Geometry: final body of the model. Coordinates: model frame, mm. A direction names the side the tool comes from. Round coordinates to 2 decimals unless told otherwise and drop trailing zeros. Write each loop counter-clockwise with the first axis right and the second up, starting at its lowest first coordinate (ties: lowest second). Pieces come first, ordered by that corner, then holes. Notation, with made-up numbers: (84.5, 2.25) -> (116.5, 2.25) arc R10 cw to (116.5, 7.25) -> close; hole circle Ø3 at (-37, -24.75). An arc over 180 degrees is marked (long way). Use one line per item in the form item = value. Start each with the question number.
1. Cut plane C-C, the plane x = -10.65. Return the cut outline in (y, z).
2. Draft query along Y for faces 1 (the face through (9.65, 7.24, 17.37)), 2 (the face through (0, 9.3, 17)), 3 (the face through (0, 0, 0)), 4 (the face through (0, 16, 18)). Return one class per face: pulls with the +Y half, pulls with the -Y half, needs draft (parallel to the pull), parting line crosses it, or undercut.
3. Line query: L1, parallel to X at y = 7.25, z = -10; L2, parallel to Z at x = 8.5, y = 21.75; L3, parallel to Y at x = -10.65, z = 19.55. Output: solid intervals per line, ascending.
4. Pin query (flat end, axial travel): pin 1 Ø2.5 at (x, y) = (-10.65, 7.2) entering from +Z; pin 2 Ø3 at (x, z) = (-5.5, -4.5) entering from +Y; pin 3 Ø1.2 at (x, y) = (-11.5, 10.5) entering from -Z. Return the tip coordinate at first contact, or that it passes through.
5. Cut plane A-A, the plane y = 7.2. Return the cut outline in (x, z).
6. Reachability of faces 5 (the face through (9.49, 12.686, -18.817)), 6 (the face through (-9.696, 7.5, 17.368)), 7 (the face through (0, 14, -17.2)) from +Z, -Z, +X, -X, +Y, -Y: full face, straight path, thin tool, end or side. Return the list, or none.
7. Cut plane B-B, the plane z = -13. Return the cut outline in (x, y), plus the area to 3 significant figures.
8. Cut plane D-D, the plane y = 18.5. Return the cut outline in (x, z), plus the area to 3 significant figures.
```python
from build123d import *

# Parameters (mm, degrees)
SKETCH_3_W           = 36
SKETCH_3_H           = 50
EXTRUDE_1_DEPTH      = 24
SKETCH_4_W           = 24.8
SKETCH_4_H           = 31.8
CUT_EXTRUDE_1_DEPTH  = 19.7
SKETCH_5_W           = 14
SKETCH_5_H           = 2.2
CUT_EXTRUDE_3_DEPTH  = 19.7
SKETCH_6_W           = 18.5
SKETCH_6_H           = 3.8
CUT_EXTRUDE_4_DEPTH  = 14.7
SKETCH_7_W           = 24.8
SKETCH_7_H           = 24.280407208
CUT_EXTRUDE_5_DEPTH  = 2
SKETCH_8_R           = 2
CUT_EXTRUDE_6_DEPTH  = 6.4
SKETCH_9_R           = 1
CUT_EXTRUDE_7_DEPTH  = 6.4
SKETCH_10_R          = 2
CUT_EXTRUDE_8_DEPTH  = 7.4
SKETCH_11_R          = 1
CUT_EXTRUDE_9_DEPTH  = 7.4
SKETCH_14_W          = 47.693248889
SKETCH_14_H          = 41.94352182
CUT_EXTRUDE_12_DEPTH = 4
SKETCH_16_W          = 69.166934332
SKETCH_16_H          = 39.422219991
CUT_EXTRUDE_13_DEPTH = 5
CUT_EXTRUDE_17_DEPTH = 19.7
SKETCH_19_W          = 18.9
SKETCH_19_H          = 2.1
CUT_EXTRUDE_18_DEPTH = 12.7
SKETCH_20_W          = 25.2
SKETCH_20_H          = 38.217614171
CUT_EXTRUDE_19_DEPTH = 2


with BuildPart() as part:
    # 草图3 → 凸台-拉伸1 (new body)
    with BuildSketch(Plane(origin=(0, 0, 0), x_dir=(1, 0, 0), z_dir=(0, 1, 0))):
        Rectangle(SKETCH_3_W, SKETCH_3_H)
    extrude(amount=EXTRUDE_1_DEPTH)

    # 草图4 → 切除-拉伸1 (cut)
    with BuildSketch(Plane(origin=(0, 24, 0), x_dir=(1, 0, 0), z_dir=(0, 1, 0))):
        Rectangle(SKETCH_4_W, SKETCH_4_H)
    extrude(amount=-CUT_EXTRUDE_1_DEPTH, mode=Mode.SUBTRACT)

    # 草图5 → 切除-拉伸3 (cut)
    with BuildSketch(Plane(origin=(0, 24, 0), x_dir=(1, 0, 0), z_dir=(0, 1, 0))):
        with Locations((0, 15.9)):
            Rectangle(SKETCH_5_W, SKETCH_5_H)
    extrude(amount=-CUT_EXTRUDE_3_DEPTH, mode=Mode.SUBTRACT)

    # 草图6 → 切除-拉伸4 (cut)
    with BuildSketch(Plane(origin=(0, 24, 0), x_dir=(1, 0, 0), z_dir=(0, 1, 0))):
        with Locations((0, -15.9)):
            Rectangle(SKETCH_6_W, SKETCH_6_H)
    extrude(amount=-CUT_EXTRUDE_4_DEPTH, mode=Mode.SUBTRACT)

    # 草图7 → 切除-拉伸5 (cut)
    with BuildSketch(Plane(origin=(0, 24, 0), x_dir=(1, 0, 0), z_dir=(0, 1, 0))):
        with Locations((0, -25)):
            Rectangle(SKETCH_7_W, SKETCH_7_H)
    extrude(amount=-CUT_EXTRUDE_5_DEPTH, mode=Mode.SUBTRACT)

    # 草图8 → 切除-拉伸6 (cut)
    with BuildSketch(Plane.XY.offset(25)):
        with Locations((10.65, 7.2)):
            Circle(SKETCH_8_R)
        with Locations((-10.65, 7.2)):
            Circle(SKETCH_8_R)
    extrude(amount=-CUT_EXTRUDE_6_DEPTH, mode=Mode.SUBTRACT)

    # 草图9 → 切除-拉伸7 (cut)
    with BuildSketch(Plane.XY.offset(18.6)):
        with Locations((10.65, 7.2)):
            Circle(SKETCH_9_R)
        with Locations((-10.65, 7.2)):
            Circle(SKETCH_9_R)
    extrude(amount=-CUT_EXTRUDE_7_DEPTH, mode=Mode.SUBTRACT)

    # 草图10 → 切除-拉伸8 (cut)
    with BuildSketch(Plane(origin=(0, 0, -25), x_dir=(-1, 0, 0), z_dir=(0, 0, -1))):
        with Locations((-10.565, 11)):
            Circle(SKETCH_10_R)
        with Locations((10.56, 11)):
            Circle(SKETCH_10_R)
    extrude(amount=-CUT_EXTRUDE_8_DEPTH, mode=Mode.SUBTRACT)

    # 草图11 → 切除-拉伸9 (cut)
    with BuildSketch(Plane(origin=(0, 0, -17.6), x_dir=(-1, 0, 0), z_dir=(0, 0, -1))):
        with Locations((10.56, 11)):
            Circle(SKETCH_11_R)
        with Locations((-10.565, 11)):
            Circle(SKETCH_11_R)
    extrude(amount=-CUT_EXTRUDE_9_DEPTH, mode=Mode.SUBTRACT)

    # 草图14 → 切除-拉伸12 (cut)
    with BuildSketch(Plane.XY.offset(25)):
        with Locations((-2.653720185, 12.393348568)):
            Rectangle(SKETCH_14_W, SKETCH_14_H)
    extrude(amount=-CUT_EXTRUDE_12_DEPTH, mode=Mode.SUBTRACT)

    # 草图16 → 切除-拉伸13 (cut)
    with BuildSketch(Plane(origin=(0, 0, -25), x_dir=(-1, 0, 0), z_dir=(0, 0, -1))):
        with Locations((0.858826259, 12.588310345)):
            Rectangle(SKETCH_16_W, SKETCH_16_H)
    extrude(amount=-CUT_EXTRUDE_13_DEPTH, mode=Mode.SUBTRACT)

    # 草图18 → 切除-拉伸17 (cut)
    with BuildSketch(Plane(origin=(0, 24, 0), x_dir=(1, 0, 0), z_dir=(0, 1, 0))):
        Polygon((-12.6, -16.1), (12.6, -16.1), (12.6, 16.1), (7.2, 16.1), (7.2, 17.2), (-7.2, 17.2), (-7.2, 16.1), (-12.6, 16.1), align=None)
    extrude(amount=-CUT_EXTRUDE_17_DEPTH, mode=Mode.SUBTRACT)

    # 草图19 → 切除-拉伸18 (cut)
    with BuildSketch(Plane(origin=(0, 22, 0), x_dir=(1, 0, 0), z_dir=(0, 1, 0))):
        with Locations((0, -16.95)):
            Rectangle(SKETCH_19_W, SKETCH_19_H)
    extrude(amount=-CUT_EXTRUDE_18_DEPTH, mode=Mode.SUBTRACT)

    # 草图20 → 切除-拉伸19 (cut)
    with BuildSketch(Plane(origin=(0, 24, 0), x_dir=(1, 0, 0), z_dir=(0, 1, 0))):
        with Locations((0, -3.008807086)):
            Rectangle(SKETCH_20_W, SKETCH_20_H)
    extrude(amount=-CUT_EXTRUDE_19_DEPTH, mode=Mode.SUBTRACT)


solid = part.part
```
Outcome:
q1.outline = (0, -20) -> (9, -20) -> (9, -17.6) -> (10, -17.6) -> (10, -16.1) -> (4.3, -16.1) -> (4.3, 16.1) -> (6.2, 16.1) -> (6.2, 18.6) -> (5.2, 18.6) -> (5.2, 21) -> (0, 21) -> close; (8.2, 16.1) -> (22, 16.1) -> (22, 21) -> (9.2, 21) -> (9.2, 18.6) -> (8.2, 18.6) -> close; (12, -17.6) -> (13, -17.6) -> (13, -20) -> (24, -20) -> (24, -16.1) -> (12, -16.1) -> close
q2.face_1 = undercut
q2.face_2 = pulls with the +Y half
q2.face_3 = pulls with the -Y half
q2.face_4 = needs draft
q3.L1 = -18 to -12.6, 12.6 to 18
q3.L2 = -20 to -16.1, 18 to 21
q3.L3 = 0 to 5.2, 9.2 to 22
q4.pin_1 = 18.6
q4.pin_2 = 4.3
q4.pin_3 = -17.6
q5.outline = (-18, -20) -> (18, -20) -> (18, 21) -> (12.65, 21) -> (12.65, 18.6) -> (11.65, 18.6) -> (11.65, 16.1) -> (12.6, 16.1) -> (12.6, -16.1) -> (7.2, -16.1) -> (7.2, -17.2) -> (-7.2, -17.2) -> (-7.2, -16.1) -> (-12.6, -16.1) -> (-12.6, 16.1) -> (-11.65, 16.1) -> (-11.65, 18.6) -> (-12.65, 18.6) -> (-12.65, 21) -> (-18, 21) -> close; (-9.65, 16.1) -> (9.65, 16.1) -> (9.65, 18.6) -> (8.65, 18.6) -> (8.65, 21) -> (-8.65, 21) -> (-8.65, 18.6) -> (-9.65, 18.6) -> close
q6.face_5 = -Z
q6.face_6 = +Z
q6.face_7 = +Y
q7.outline = (-18, 0) -> (18, 0) -> (18, 24) -> (12.6, 24) -> (12.6, 4.3) -> (-12.6, 4.3) -> (-12.6, 24) -> (-18, 24) -> close
q7.area = 368 mm^2
q8.outline = (-18, -20) -> (18, -20) -> (18, 21) -> (-18, 21) -> close; hole (-12.6, -16.1) -> (-7.2, -16.1) -> (-7.2, -17.2) -> (7.2, -17.2) -> (7.2, -16.1) -> (12.6, -16.1) -> (12.6, 16.1) -> (9.45, 16.1) -> (9.45, 18) -> (-9.45, 18) -> (-9.45, 16.1) -> (-12.6, 16.1) -> close
q8.area = 613 mm^2
